Verification items for the finished model (mm, model axes). A direction names the side the tool comes from. Coordinates: 2 decimals unless noted, no trailing zeros. Order: outer loops, then holes, each group sorted by start corner. A loop starts at its lowest first (then second) coordinate and runs counter-clockwise, first axis right, second up. Notation, with made-up numbers: M -37.75,40.5 L 20.25,40.5 A35 cw 20.25,76.5 Z; hole C 34.25,26.25 d10. An arc over 180 degrees is marked long. Return JSON: item names as keys, results as strings. Group by question number.
Q1. Section check B-B, the plane y = -13.5. Enter the section's corners in (x, z).
Q2. Thickness scan on probe 1 along Z at (x, y) = (-41, -5.75); probe 2 along Z at (x, y) = (-41.5, -14.5); probe 3 along Y at (x, z) = (-14, -38). Record the ranges inside material, lowest first.
Q3. Mould release check, pull along Y, two halves, no side actions. Record for faces 4 (the face through (-20, -10, 53)), 5 (the face through (-23, 0, 22)), 6 (the face through (-14, -23, -32)): pulls with the +Y half, pulls with the -Y half, needs draft (parallel to the pull), parting line crosses it, or undercut.
Q4. Section check C-C, the plane x = -38.5. Enter the section's corners in (y, z).
Q5. Section check D-D, the plane x = -14. Enter the section's corners in (y, z).
Q6. Section check A-A, the plane z = 5. Enter the section's corners in (x, y).
Q7. Go/stop test with flat-tipped pins: pin 1 Ø1.5 at (x, y) = (-43.5, -9) entering from +Z; pin 2 Ø4 at (y, z) = (-13, 52.5) entering from +X; pin 3 Ø4 at (y, z) = (-15.5, 8) entering from -X. Record where each tip stops, or that it passes through.
Q8. Access from +Z, -Z, +X, -X, +Y, -Y to the whole of each face (thin tool, end or side, straight path). Record for faces 1 (the face through (-14, -14, -32)), 2 (the face through (-8.924, -3.741, -15.776)), 3 (the face through (-29, -14, -38)).
from build123d import *

# Parameters (mm, degrees)
F0_W      = 46
F0_H      = 43
F0_R      = 1
F1_DEPTH  = 25
F4_R      = 7
F3_R      = 17
F3_R_2    = 1
F5_DEPTH  = 4
F7_W      = 21
F7_H      = 19.5
F8_DEPTH  = 8
F10_DEPTH = 7
F11_R     = 11
F12_DEPTH = 32
F13_R     = 3
F14_DEPTH = 11.5


with BuildPart() as f1:
    # F0 (on Front) → F1 (new body)
    with BuildSketch(Plane.XZ):
        with Locations((-23, 21.5)):
            Rectangle(F0_W, F0_H)
        with Locations((-41, 5)):
            Circle(F0_R, mode=Mode.SUBTRACT)
        with Locations((-41, 36)):
            Circle(F0_R, mode=Mode.SUBTRACT)
        with Locations((-10, 36)):
            Circle(F0_R, mode=Mode.SUBTRACT)
    extrude(amount=F1_DEPTH)

    # F4
    f4_edges = [f1.edges().sort_by_distance(p)[0] for p in [
        (0, -12.5, 43),
    ]]
    fillet(f4_edges, radius=F4_R)

    # F3 (on offset) → F5 (join)
    with BuildSketch(Plane(origin=(0, -4, 0), x_dir=(-1, 0, 0), z_dir=(0, 1, 0))):
        with Locations((10, 36)):
            Circle(F3_R)
        with Locations((10, 36)):
            Circle(F3_R_2, mode=Mode.SUBTRACT)
    extrude(amount=-F5_DEPTH)

    # F7 (on offset) → F8 (join)
    with BuildSketch(Plane(origin=(0, -10, 0), x_dir=(-1, 0, 0), z_dir=(0, 1, 0))):
        with Locations((20.5, 52.75)):
            Rectangle(F7_W, F7_H)
    extrude(amount=-F8_DEPTH)

    # F9 (on face) → F10 (join)
    with BuildSketch(Plane(origin=(-46, 0, 0), x_dir=(0, -1, 0), z_dir=(-1, 0, 0))):
        with BuildLine():
            Line((20, 43), (5, 43))
            ThreePointArc((5, 43), (12.5, 35.5), (20, 43))
        make_face()
        with BuildLine():
            ThreePointArc((20, 43), (12.5, 50.5), (5, 43))
            Line((5, 43), (20, 43))
        make_face()
    extrude(amount=F10_DEPTH)

    # F11 (on face) → F12 (join)
    with BuildSketch(Plane(origin=(0, 0, 0), x_dir=(1, 0, 0), z_dir=(0, 0, -1))):
        with Locations((-14, 13.5)):
            Circle(F11_R)
    extrude(amount=F12_DEPTH)

    # F13 (on face) → F14 (join)
    with BuildSketch(Plane(origin=(0, 0, -32), x_dir=(1, 0, 0), z_dir=(0, 0, -1))):
        with BuildLine():
            ThreePointArc((-21.5498344353, 5.5), (-25, 13.5), (-21.5498344353, 21.5))
            Line((-21.5498344353, 21.5), (-29, 21.5))
            Line((-29, 21.5), (-29, 5.5))
            Line((-29, 5.5), (-21.5498344353, 5.5))
        make_face()
        with BuildLine():
            Line((-6, 5.9501655647), (-6, 21.0498344353))
            ThreePointArc((-6, 21.0498344353), (-6.2218254069, 21.2781745931), (-6.4501655647, 21.5))
            Line((-6.4501655647, 21.5), (-21.5498344353, 21.5))
            ThreePointArc((-21.5498344353, 21.5), (-25, 13.5), (-21.5498344353, 5.5))
            Line((-21.5498344353, 5.5), (-6.4501655647, 5.5))
            ThreePointArc((-6.4501655647, 5.5), (-6.2218254069, 5.7218254069), (-6, 5.9501655647))
        make_face()
        with Locations((-14, 13.5)):
            Circle(F13_R, mode=Mode.SUBTRACT)
        with BuildLine():
            Line((-6, 5.5), (-6, 5.9501655647))
            ThreePointArc((-6, 5.9501655647), (-6.2218254069, 5.7218254069), (-6.4501655647, 5.5))
            Line((-6.4501655647, 5.5), (-6, 5.5))
        make_face()
        with BuildLine():
            ThreePointArc((-6.4501655647, 21.5), (-6.2218254069, 21.2781745931), (-6, 21.0498344353))
            Line((-6, 21.0498344353), (-6, 21.5))
            Line((-6, 21.5), (-6.4501655647, 21.5))
        make_face()
    extrude(amount=F14_DEPTH)


solid = f1.part
Numbers:
{
 "1": {"outline": "M -53,35.57 L -46,35.57 L -46,0 L -25,0 L -25,-32 L -29,-32 L -29,-43.5 L -17,-43.5 L -17,-32 L -11,-32 L -11,-43.5 L -6,-43.5 L -6,-32 L -3,-32 L -3,0 L 0,0 L 0,36 A7 ccw -7,43 L -10,43 L -10,62.5 L -31,62.5 L -31,43 L -46,43 L -46,50.43 L -53,50.43 Z; hole C -41,5 d2; hole C -41,36 d2; hole C -10,36 d2"},
 "2": {"probe 1": "z = 0 to 4, 6 to 35, 37 to 43", "probe 2": "z = 0 to 4.13, 5.87 to 35.13, 36.87 to 43", "probe 3": "y = -21.5 to -16.5, -10.5 to -5.5"},
 "3": {"face 4": "undercut", "face 5": "pulls with the +Y half", "face 6": "needs draft"},
 "4": {"outline": "M -25,0 L 0,0 L 0,43 L -25,43 Z"},
 "5": {"outline": "M -25,0 L -24.5,0 L -24.5,-32 L -21.5,-32 L -21.5,-43.5 L -16.5,-43.5 L -16.5,-32 L -10.5,-32 L -10.5,-43.5 L -5.5,-43.5 L -5.5,-32 L -2.5,-32 L -2.5,0 L 0,0 L 0,43 L -4,43 L -4,52.52 L -8,52.52 L -8,43 L -10,43 L -10,62.5 L -18,62.5 L -18,43 L -25,43 Z"},
 "6": {"outline": "M -46,-25 L -42,-25 L -42,0 L -46,0 Z; M -40,-25 L 0,-25 L 0,0 L -40,0 Z"},
 "7": {"pin 1": "stops at z = 43", "pin 2": "stops at x = -10", "pin 3": "stops at x = -46"},
 "8": {"face 1": "-Z", "face 2": "none", "face 3": "-Z, -X, +Y, -Y"}
}
